```python
from build123d import *

# Parameters (mm, degrees)
SKETCH1_W           = 20
SKETCH1_H           = 50
SKETCH1_W_2         = 30
SKETCH1_H_2         = 20
BOSS_EXTRUDE1_DEPTH = 3
SKETCH3_R           = 2.75
CUT_EXTRUDE1_DEPTH  = 3


with BuildPart() as part:
    # Sketch1 → Boss-Extrude1 (new body)
    with BuildSketch(Plane(origin=(0, 0, 0), x_dir=(1, 0, 0), z_dir=(0, 1, 0))):
        with Locations((10, -25)):
            Rectangle(SKETCH1_W, SKETCH1_H)
        with Locations((35, -10)):
            Rectangle(SKETCH1_W_2, SKETCH1_H_2)
    extrude(amount=BOSS_EXTRUDE1_DEPTH)

    # Sketch3 → Cut-Extrude1 (cut)
    with BuildSketch(Plane(origin=(0, 3, 0), x_dir=(1, 0, 0), z_dir=(0, 1, 0))):
        with Locations((10, -38)):
            Circle(SKETCH3_R)
        with Locations((10, -23)):
            Circle(SKETCH3_R)
        with Locations((38, -10)):
            Circle(SKETCH3_R)
        with Locations((23, -10)):
            Circle(SKETCH3_R)
    extrude(amount=-CUT_EXTRUDE1_DEPTH, mode=Mode.SUBTRACT)


solid = part.part
```
Part model, mm, in its own coordinate system. A direction names the side the tool comes from. Round coordinates to 2 decimals unless told otherwise and drop trailing zeros. Write each loop counter-clockwise with the first axis right and the second up, starting at its lowest first coordinate (ties: lowest second). Pieces come first, ordered by that corner, then holes. Notation, with made-up numbers: M 68.25,67 L 109.25,67 A28 ccw 109.25,86 Z; hole C -24.75,-26.75 d9. An arc over 180 degrees is marked long. One line per question, with ' | ' between items.
(1) Probe line 1 along X through (y, z) = (1.4, 38); line 2 along X through (y, z) = (1.05, 11). List the from-to ranges inside material, lowest first.
Answer key:
line 1: x = 0 to 7.25, 12.75 to 20 | line 2: x = 0 to 20.44, 25.56 to 35.44, 40.56 to 50
(2) Saw through at D-D on y = 1.35. Write the cut outline in (x, z), then the cut area to 3 significant figures.
Answer key:
outline: M 0,0 L 50,0 L 50,20 L 20,20 L 20,50 L 0,50 Z; hole C 10,23 d5.5; hole C 10,38 d5.5; hole C 23,10 d5.5; hole C 38,10 d5.5 | area: 1,500 mm^2
(3) Saw through at A-A on z = 23. Write the cut outline in (x, y).
Answer key:
outline: M 0,0 L 7.25,0 L 7.25,3 L 0,3 Z; M 12.75,0 L 20,0 L 20,3 L 12.75,3 Z
(4) Saw through at B-B on x = 23. Write the cut outline in (y, z), then the cut area to 3 significant figures.
Answer key:
outline: M 0,0 L 3,0 L 3,7.25 L 0,7.25 Z; M 0,12.75 L 3,12.75 L 3,20 L 0,20 Z | area: 43.5 mm^2
(5) 3-axis set-ups, long thin cutter, end or side, ignore diameter. For faces 4 (the face through (35, 1, 20)), 5 (the face through (25, 1, 0)): which of +Z, -Z, +X, -X, +Y, -Y reach the whole face in a straight line?
Answer key:
face 4: +Z, +X, +Y, -Y | face 5: -Z, +X, -X, +Y, -Y
(6) Two-plate mould, pull along X, no slides. Class faces 1 (the face through (9.642, 1.521, 20.273)), 2 (the face through (10, 1, 50)), 3 (the face through (50, 1, 10)): released by +X, released by -X, zero draft, split by the parting line, or undercut.
Answer key:
face 1: undercut | face 2: zero draft | face 3: released by +X
(7) Saw through at C-C on z = 10. Write the cut outline in (x, y), then the cut area to 3 significant figures.
Answer key:
outline: M 0,0 L 20.25,0 L 20.25,3 L 0,3 Z; M 25.75,0 L 35.25,0 L 35.25,3 L 25.75,3 Z; M 40.75,0 L 50,0 L 50,3 L 40.75,3 Z | area: 117 mm^2
(8) Pin check, flat tip, straight feed: pin 1 (7 mm diameter, centred on x = 10, z = 23, fed in from -Y). Stop position of the tip, or through.
Answer key:
pin 1: stops at y = 0
